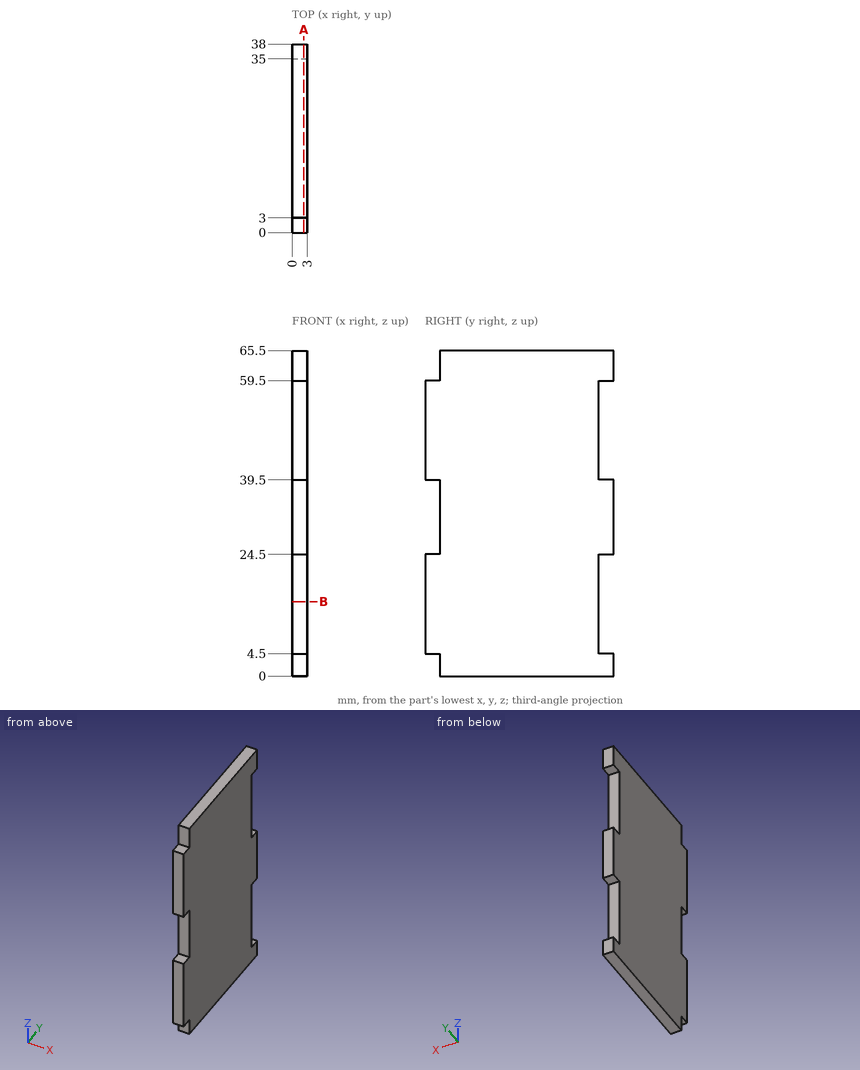
For this review, use the dimensioned drawing (mm, ordinates from the lowest corner) and the shaded views. Coordinates: 2 decimals unless noted, no trailing zeros. Write each loop counter-clockwise with the first axis right and the second up, starting at its lowest first coordinate (ties: lowest second). Pieces come first, ordered by that corner, then holes. Notation, with made-up numbers: (-28.75, 65) - (-3.75, 65) arc R7 cw to (-3.75, 76) - close; hole circle Ø7 at (4.25, -38.75). An arc over 180 degrees is marked (long way). Answer as a JSON object with one key per item and string values. Group by question number.
1. Clearance check with flat-ended pins moving along their axes: pin 1 Ø1.5 at (x, y) = (1, 1) entering from +Z; pin 2 Ø10 at (y, z) = (13, 49) entering from -X; pin 3 Ø0.9 at (x, z) = (2, 33) entering from -Y; pin 4 Ø0.9 at (x, y) = (2, 1.5) entering from -Z. State where each tip first meets the part, or that it passes through.
2. Add section A-A (x = 2.35). Give the boundary of the cut face in (y, z), plus the area to 3 significant figures.
3. To check wall thickness, follow probe 1 along Y at (x, z) = (1.05, 14.5); probe 2 along Y at (x, z) = (2.1, 26). State the ranges of each line that lie inside material, in increasing order.
4. Add section B-B (z = 15). Give the boundary of the cut face in (x, y).
Findings:
{
 "1": {"pin 1": "z = 59.5", "pin 2": "x = 0", "pin 3": "y = 3", "pin 4": "z = 4.5"},
 "2": {"outline": "(0, 4.5) - (3, 4.5) - (3, 0) - (38, 0) - (38, 4.5) - (35, 4.5) - (35, 24.5) - (38, 24.5) - (38, 39.5) - (35, 39.5) - (35, 59.5) - (38, 59.5) - (38, 65.5) - (3, 65.5) - (3, 59.5) - (0, 59.5) - (0, 39.5) - (3, 39.5) - (3, 24.5) - (0, 24.5) - close", "area": "2,290 mm²"},
 "3": {"probe 1": "0 to 35", "probe 2": "3 to 38"},
 "4": {"outline": "(0, 0) - (3, 0) - (3, 35) - (0, 35) - close"}
}
